Autodesk Inventor part; units mm, degrees
ref_plane "YZ Plane" through (0, 0, 0) normal (1, 0, 0) x (0, 1, 0)
ref_plane "XZ Plane" through (0, 0, 0) normal (0, 1, 0) x (-1, 0, 0)
ref_plane "XY Plane" through (0, 0, 0) normal (0, 0, 1) x (1, 0, 0)
sketch "Náčrt1" plane through (0, 0, 0) normal (0, 0, 1) x (1, 0, 0)
  circle A0 centre (0, 0) radius 2.5
  dimension "d0" = 5
extrude "Vysunutí1" add sketch "Náčrt1" along normal mid plane 251
sketch "Náčrt2" plane through (0, 0, 125.5) normal (0, 0, 1) x (1, 0, 0)
  point P0 (0, 0)
  point P1 (0, 0)
hole "Díra1" at (0, 0, 125.5) direction (0, 0, -1) diameter 2.459 depth 10 tip angle 118
mirror "Zrcadlit1" about plane through (0, 0, 0) normal (0, 0, 1) of "Díra1"
properties part number "lifter_rod" material "Hliník 6061"
The model under review builds one solid part; all positions refer to its coordinate system, in mm. Round coordinates to 2 decimals unless told otherwise and drop trailing zeros. Loops run counter-clockwise (first coordinate to the right, second up) from the corner with the lowest first, then second, coordinate; pieces in that order, holes last. Notation, with made-up numbers: M 45,6 L 99,6 A20 cw 99,33 Z; hole C -29,20.5 d8. An arc over 180 degrees is marked long. Answer as CSV lines item,"result".
1. We need section A-A (z = 53). Give the boundary of the cut face in (x, y).
Outcome:
outline,"C 0,0 d5"
2. To check wall thickness, follow L1, parallel to Y at x = 0, z = 118.75; L2, parallel to X at y = -2.2, z = 88; L3, parallel to Z at x = -0.7, y = -0.25. State the ranges of each line that lie inside material, in increasing order. Write a range as [from, to].
Outcome:
L1,"y = [-2.5, -1.23], [1.23, 2.5]"
L2,"x = [-1.19, 1.19]"
L3,"z = [-115.21, 115.21]"
3. Insertion check: pin 1 Ø1.5 at (x, z) = (-1.5, -9.5) entering from +Y; pin 2 Ø2 at (x, y) = (0, 0) entering from +Z; pin 3 Ø1.5 at (y, z) = (-1.5, 96) entering from -X. Each pin has a flat end and moves straight along its axis. Give the tip position at first contact, or say it passes through.
Outcome:
pin 1,"stops at y = 2.38"
pin 2,"stops at z = 115.36"
pin 3,"stops at x = -2.38"
